Work out the finished part from the listing and answer in its coordinate system (mm). Round coordinates to 2 decimals unless told otherwise and drop trailing zeros. Loops run counter-clockwise (first coordinate to the right, second up) from the corner with the lowest first, then second, coordinate; pieces in that order, holes last. Notation, with made-up numbers: (-28, 64) -> (-24, 64) arc R23 ccw to (-24, 81) -> close; hole circle Ø7 at (-10.5, 86). An arc over 180 degrees is marked (long way). Use one line per item in the form item = value.
```python
from build123d import *

# Parameters (mm, degrees)
F1_DEPTH = 254
F3_D     = 3.5814
F3_DEPTH = 19.05
F3_TIP   = 1.0759611105
F4_DEPTH = 10.16
F5_DEPTH = 10.16


with BuildPart() as f1:
    # F0 (on Front) → F1 (new body)
    with BuildSketch(Plane.XZ):
        Polygon((49.1248931152, -56.7675527828), (-39.7751068848, -57.0361235134), (48.4362465841, -57.0361235134), (49.1248931152, -57.0361235134), align=None)
        with BuildLine():
            ThreePointArc((49.1248931152, 25.5138764866), (18.3482789064, -30.4863082116), (-39.7751068848, -57.0361235134))
            Line((-39.7751068848, -57.0361235134), (49.1248931152, -56.7675527828))
            Line((49.1248931152, -56.7675527828), (49.1248931152, 25.5138764866))
        make_face()
        Polygon((48.4362465841, -57.0361235134), (-39.7751068848, -57.0361235134), (-39.7751068848, -69.7361235134), (61.8248931152, -69.7361235134), (61.8248931152, -57.0361235134), (55.4748931152, -57.0361235134), (49.1248931152, -57.0361235134), align=None)
        Polygon((49.1248931152, 25.5138764866), (49.1248931152, -56.7675527828), (49.1248931152, -57.0361235134), (55.4748931152, -57.0361235134), (61.8248931152, -57.0361235134), (61.8248931152, 25.5138764866), align=None)
    extrude(amount=F1_DEPTH)

    # F3
    with Locations(Plane.YZ.offset(61.8248931152)):
        with Locations((-228.5564392805, -22.1111235134), (-180.5504392805, -22.1111235134), (-132.5444392805, -22.1111235134), (-84.5384392805, -22.1111235134), (-36.5324392805, -22.1111235134)):
            Hole(F3_D / 2, depth=F3_DEPTH)
            with Locations((0, 0, -(F3_DEPTH + F3_TIP / 2))):  # 118° drill point
                Cone(0, F3_D / 2, F3_TIP, mode=Mode.SUBTRACT)

    # F4 (cut): a face of the model
    f4_faces = [f1.faces().sort_by_distance(p)[0] for p in [
        (61.8248931152, -126.9884327642, -22.1111235134),
    ]]
    extrude(f4_faces, amount=-F4_DEPTH, mode=Mode.SUBTRACT)

    # F5 (cut): a face of the model
    f5_faces = [f1.faces().sort_by_distance(p)[0] for p in [
        (5.9448931152, -127, -69.7361235134),
    ]]
    extrude(f5_faces, amount=-F5_DEPTH, mode=Mode.SUBTRACT)


solid = f1.part
```
(1) Find section A-A, the plane y = -57.5. Write down the section's boundary in (x, z), then the cut area to 3 significant figures.
Completed:
outline = (-39.78, -59.58) -> (51.66, -59.58) -> (51.66, 25.51) -> (49.12, 25.51) arc R101.6 cw to (-39.78, -57.04) -> close
area = 2,450 mm2
(2) Consider L1, parallel to X at y = -102, z = 2; L2, parallel to X at y = -122.5, z = -36; L3, parallel to Z at x = 12, y = -16. Determine where each line is inside the solid, lowest interval first.
Completed:
L1 = 41.74 to 51.66
L2 = 11.89 to 51.66
L3 = -59.58 to -35.91
(3) Find section B-B, the plane x = 20.5. Write down the section's boundary in (y, z).
Completed:
outline = (-254, -59.58) -> (0, -59.58) -> (0, -28.43) -> (-254, -28.43) -> close
(4) Find section C-C, the plane z = 13. Write down the section's boundary in (x, y), then the cut area to 3 significant figures.
Completed:
outline = (45.98, -254) -> (51.66, -254) -> (51.66, 0) -> (45.98, 0) -> close
area = 1,440 mm2
(5) Given P1, Ø3, axis at y = -36.53, z = -22.11, coming from the -X side; P2, Ø1, axis at y = -129.5, z = -11, coming from the -X side; P3, Ø10, axis at y = -212.5, z = -1.5, coming from the -X side, each flat-ended and moving along its own axis, determine where each tip first touches the part or whether it passes through.
Completed:
P1 = 25.08
P2 = 34.34
P3 = 37.39
